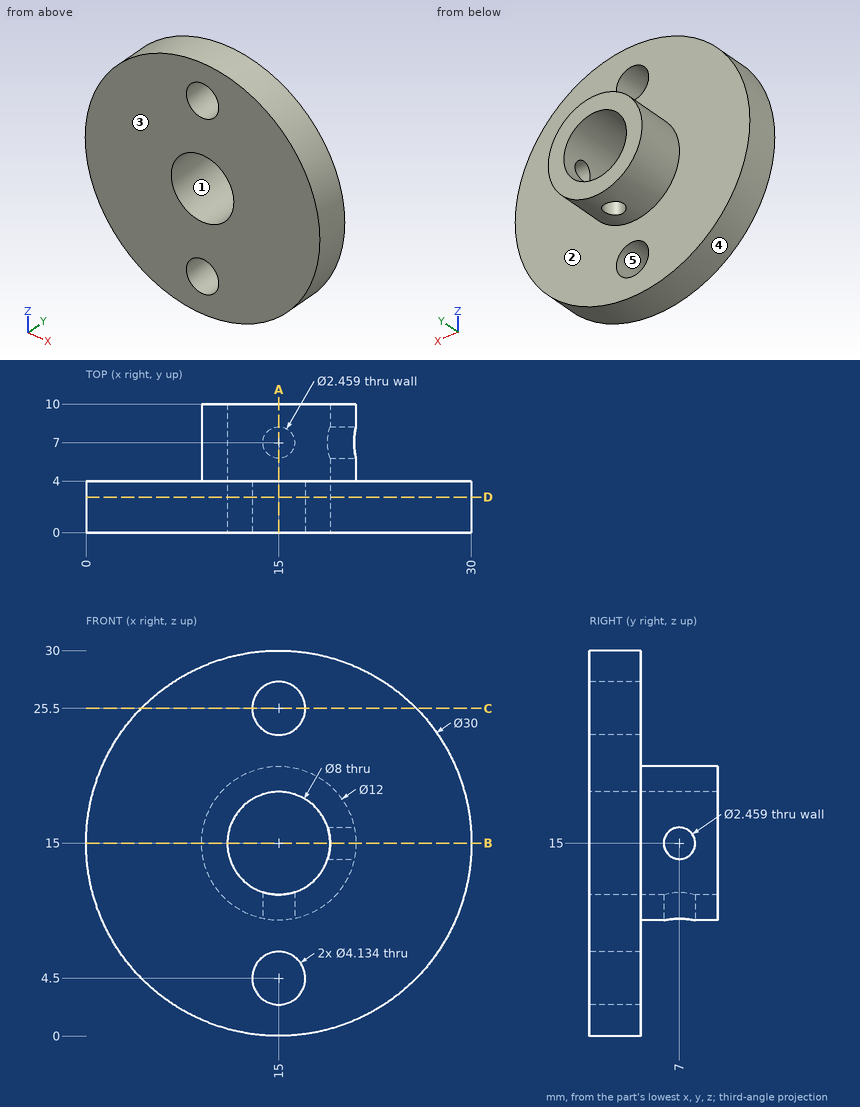
Can you work these out from the drawing? Everything is in mm from the part's minimum corner. A direction names the side the tool comes from. Round coordinates to 2 decimals unless told otherwise and drop trailing zeros. Loops run counter-clockwise (first coordinate to the right, second up) from the corner with the lowest first, then second, coordinate; pieces in that order, holes last. Notation, with made-up numbers: (14, 55) - (41, 55) arc R11 ccw to (41, 67) - close; hole circle Ø6 at (-39.5, 81). An arc over 180 degrees is marked (long way). Write item = value, one per line. Start each with the question number.
(1) For the marked faces 1 and 2, which set-ups out of +Z, -Z, +X, -X, +Y, -Y let a thin tool reach every point of the face, with its end or its side?
(2) If we section it at C-C (z = 25.5): Please give me the cut outline in (x, y), and give its area (3 significant figures).
(3) If I drill on probe 1 along Z at (x, y) = (15, 1.15); probe 2 along Y at (x, z) = (19.4, 15); probe 3 along Y at (x, z) = (9, 3.5), over which ranges is the centre line in solid material (lowest first)? Write a range as [from, to].
(4) If we section it at D-D (y = 2.75): Please give me the cut outline in (x, z).
(5) For P1, Ø4, axis at y = 7, z = 24.5, coming from the -X side; P2, Ø5.5, axis at x = 15, z = 4.5, coming from the +Y side; P3, Ø13, axis at x = 15, z = 15, coming from the +Y side; P4, Ø1.5, axis at y = 7, z = 15, coming from the +X side, each with a flat end and sliding along its axis, tell me the tip position at first contact or that it passes through.
(6) If we mould it in two halves opening along Z, with no side actions, what happens to the marked faces 3, 4 and 5? For each: released by +Z, released by -Z, zero draft, split by the parting line, or undercut.
(7) If we section it at B-B (z = 15): Please give me the cut outline in (x, y).
(8) If we section it at A-A (x = 15): Please give me the cut outline in (y, z).
Ans:
q1.face_1 = +Y, -Y
q1.face_2 = +Y
q2.outline = (4.29, 0) - (12.93, 0) - (12.93, 4) - (4.29, 4) - close; (17.07, 0) - (25.71, 0) - (25.71, 4) - (17.07, 4) - close
q2.area = 69.2 mm²
q3.probe_1 = [0, 2.43], [6.57, 11], [19, 23.43], [27.57, 30]
q3.probe_2 = [0, 5.77], [8.23, 10]
q3.probe_3 = [0, 4]
q4.outline = circle Ø30 at (15, 15); hole circle Ø8 at (15, 15); hole circle Ø4.13 at (15, 4.5); hole circle Ø4.13 at (15, 25.5)
q5.P1 = through
q5.P2 = 4
q5.P3 = 10
q5.P4 = 11.07
q6.face_3 = zero draft
q6.face_4 = split by the parting line
q6.face_5 = undercut
q7.outline = (0, 0) - (11, 0) - (11, 10) - (9, 10) - (9, 4) - (0, 4) - close; (19, 0) - (30, 0) - (30, 4) - (21, 4) - (21, 5.77) - (19, 5.77) - close; (19, 8.23) - (21, 8.23) - (21, 10) - (19, 10) - close
q8.outline = (0, 0) - (4, 0) - (4, 2.43) - (0, 2.43) - close; (0, 6.57) - (4, 6.57) - (4, 9) - (5.77, 9) - (5.77, 11) - (0, 11) - close; (0, 19) - (10, 19) - (10, 21) - (4, 21) - (4, 23.43) - (0, 23.43) - close; (0, 27.57) - (4, 27.57) - (4, 30) - (0, 30) - close; (8.23, 9) - (10, 9) - (10, 11) - (8.23, 11) - close
